Read the model definition and answer for the solid it produces. Units are mm, in the model's axes. A direction names the side the tool comes from. Coordinates: 2 decimals unless noted, no trailing zeros. Order: outer loops, then holes, each group sorted by start corner. A loop starts at its lowest first (then second) coordinate and runs counter-clockwise, first axis right, second up. Notation, with made-up numbers: (23.25, -9) - (63.25, -9) arc R21 cw to (63.25, 4) - close; hole circle Ø9 at (80, 36). An arc over 180 degrees is marked (long way). Use one line per item in the form item = value.
```python
from build123d import *

# Parameters (mm, degrees)
F1_DEPTH = 3
F2_R     = 0.5
F3_R     = 0.39999


# Not quite as in the source:
# - a fillet or chamfer is up to 0.001 mm smaller than in the source, because OpenCascade refuses the exact size


with BuildPart() as f1:
    # F0 (on Front) → F1 (new body)
    with BuildSketch(Plane.XZ):
        Polygon((-7.0882368928, 3.6), (-7.0882368928, -3.6), (7.0882368928, -3.6), (7.0882368928, 3.6), (1.5882368928, 3.6), (1.5882368928, 1.6), (1.5882368928, 1.2), (1.9882368928, 1.2), (1.9882368928, 1.6), (5.0882368928, 1.6), (5.0882368928, -1.6), (-5.0882368928, -1.6), (-5.0882368928, 1.6), (-1.9882368928, 1.6), (-1.9882368928, 1.2), (-1.5882368928, 1.2), (-1.5882368928, 1.6), (-1.5882368928, 3.6), align=None)
    extrude(amount=F1_DEPTH)

    # F2
    f2_edges = [f1.edges().sort_by_distance(p)[0] for p in [
        (4.338237, 0, 3.6),
        (-4.338237, 0, 3.6),
        (-7.088237, 0, 0),
        (0, 0, -3.6),
        (7.088237, 0, 0),
        (1.588237, -1.5, 3.6),
        (-1.588237, -1.5, 3.6),
        (-4.338237, -3, 3.6),
        (-7.088237, -1.5, 3.6),
        (4.338237, -3, 3.6),
        (3.538237, -3, 1.6),
        (-3.538237, -3, 1.6),
        (3.538237, 0, 1.6),
        (-3.538237, 0, 1.6),
        (-7.088237, -3, 0),
        (7.088237, -3, 0),
        (5.088237, -3, 0),
        (-5.088237, 0, 0),
        (-7.088237, -1.5, -3.6),
        (7.088237, -1.5, -3.6),
        (5.088237, 0, 0),
        (0, 0, -1.6),
        (0, -3, -1.6),
        (0, -3, -3.6),
    ]]
    fillet(f2_edges, radius=F2_R)

    # F3 (radius 0.4 in the source; OpenCascade refuses exactly that, so slightly less here)
    f3_edges = [f1.edges().sort_by_distance(p)[0] for p in [
        (1.588237, -1.5, 1.2),
        (-1.588237, -1.5, 1.2),
    ]]
    fillet(f3_edges, radius=F3_R)


solid = f1.part
```
(1) Section B-B, the plane z = 0.25 is taken. Write down the section's boundary in (x, y), then the cut area to 3 significant figures.
Answer list:
outline = (-7.09, -2.5) arc R0.5 ccw to (-6.59, -3) - (-5.09, -3) - (-5.09, -0.5) arc R0.5 ccw to (-5.59, 0) - (-6.59, 0) arc R0.5 ccw to (-7.09, -0.5) - close; (5.09, -2.5) arc R0.5 ccw to (5.59, -3) - (6.59, -3) arc R0.5 ccw to (7.09, -2.5) - (7.09, -0.5) arc R0.5 ccw to (6.59, 0) - (5.59, 0) arc R0.5 ccw to (5.09, -0.5) - close
area = 11.6 mm2
(2) Given pin 1 Ø1 at (x, z) = (3, -1.5) entering from +Y, flat-ended and moving along its own axis, determine where the tip first touches the part or whether it passes through.
Answer list:
pin_1 = -0.01
(3) Section C-C, the plane x = 0 is taken. Write down the section's boundary in (y, z).
Answer list:
outline = (-3, -3.1) arc R0.5 ccw to (-2.5, -3.6) - (-0.5, -3.6) arc R0.5 ccw to (0, -3.1) - (0, -2.1) arc R0.5 ccw to (-0.5, -1.6) - (-2.5, -1.6) arc R0.5 ccw to (-3, -2.1) - close
(4) Which of the six approach directions +Z, -Z, +X, -X, +Y, -Y give full straight-line access (tool end or side, diameter ignored) to faces 1 (the flat face through (1.588, -1, 2)), 2 (the flat face through (0, -1, -1.6)), 3 (the flat face through (-0.1, -3, -2.7))?
Answer list:
face_1 = +Z, +Y, -Y
face_2 = +Y, -Y
face_3 = +Z, -Z, +X, -X, -Y
(5) The mould has two halves that part along Z. Classify faces 4 (the flat face through (-4, -1, 3.6)), 5 (the flat face through (-5.088, -2, 0)), 6 (the flat face through (-0.1, 0, -2.7)), 7 (the flat face through (5.088, -1, 0)): +Z half, -Z half, draft (parallel to the pull), parting line (faces both ways), or undercut.
Answer list:
face_4 = +Z half
face_5 = undercut
face_6 = draft
face_7 = undercut
(6) Straight lines are drawn through the part: L1, parallel to X at y = -0.7, z = 1.5; L2, parallel to Z at x = 5, y = -1.6; L3, parallel to X at y = -1.15, z = -0.75. For each, find the intervals that lie inside material, in ascending order.
Answer list:
L1 = -7.09 to -5.09, -1.99 to -1.6, 1.6 to 1.99, 5.09 to 7.09
L2 = -3.6 to -1.6, 1.6 to 3.6
L3 = -7.09 to -5.09, 5.09 to 7.09
(7) Section A-A, the plane x = 4.25 is taken. Write down the section's boundary in (y, z), then the cut area to 3 significant figures.
Answer list:
outline = (-3, -3.1) arc R0.5 ccw to (-2.5, -3.6) - (-0.5, -3.6) arc R0.5 ccw to (0, -3.1) - (0, -2.1) arc R0.5 ccw to (-0.5, -1.6) - (-2.5, -1.6) arc R0.5 ccw to (-3, -2.1) - close; (-3, 2.1) arc R0.5 ccw to (-2.5, 1.6) - (-0.5, 1.6) arc R0.5 ccw to (0, 2.1) - (0, 3.1) arc R0.5 ccw to (-0.5, 3.6) - (-2.5, 3.6) arc R0.5 ccw to (-3, 3.1) - close
area = 11.6 mm2
